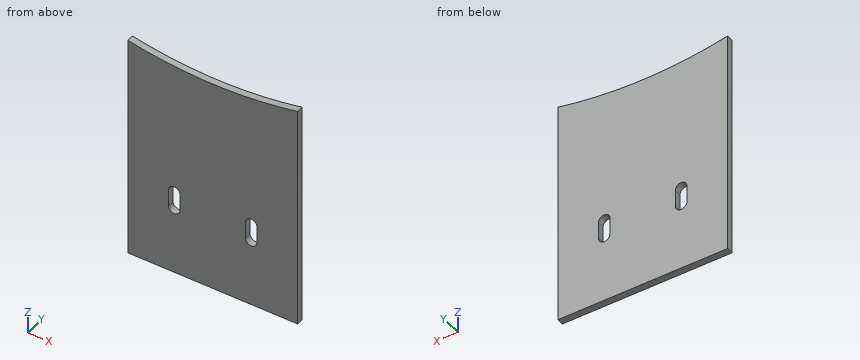
```python
from build123d import *

# Parameters (mm, degrees)
SM_BASE_FLANGE_1_DEPTH = 16


# Sheet-metal steps are written as plain solids
with BuildPart() as part:
    # Sketch 1 → 基体-法兰1 (new body)
    with BuildSketch(Plane(origin=(0, 0, 0), x_dir=(1, 0, 0), z_dir=(0, 1, 0))):
        with BuildLine():
            Line((-200, 964.992357483), (-200, 1497.5))
            Line((-200, 1497.5), (200, 1497.5))
            Line((200, 1497.5), (200, 964.992357483))
            ThreePointArc((200, 964.992357483), (0, 985.5), (-200, 964.992357483))
        make_face()
        with BuildLine():
            Line((-77, 1337), (-77, 1297))
            ThreePointArc((-77, 1297), (-90.5, 1283.5), (-104, 1297))
            Line((-104, 1297), (-104, 1337))
            ThreePointArc((-104, 1337), (-90.5, 1350.5), (-77, 1337))
        make_face(mode=Mode.SUBTRACT)
        with BuildLine():
            Line((77, 1297), (77, 1337))
            ThreePointArc((77, 1337), (90.5, 1350.5), (104, 1337))
            Line((104, 1337), (104, 1297))
            ThreePointArc((104, 1297), (90.5, 1283.5), (77, 1297))
        make_face(mode=Mode.SUBTRACT)
    extrude(amount=SM_BASE_FLANGE_1_DEPTH)


solid = part.part
```
Here's how the part is built. I have some questions about the finished solid (model axes, mm). Round coordinates to 2 decimals unless told otherwise and drop trailing zeros. Write each loop counter-clockwise with the first axis right and the second up, starting at its lowest first coordinate (ties: lowest second). Pieces come first, ordered by that corner, then holes. Notation, with made-up numbers: M 27,86.25 L 69,86.25 A11 cw 69,106.25 Z; hole C -21.5,13.5 d7. An arc over 180 degrees is marked long. Answer as CSV lines item,"result". Start each with the question number.
1. Suppose I cut it at B-B on x = 90.5. Write out the boundary of the cut face in (y, z), then the cut area to 3 significant figures.
2. I need wall thicknesses on probe 1 along X at (y, z) = (13.5, -1300.5); probe 2 along Z at (x, y) = (-13, 2); probe 3 along Z at (x, y) = (93, 6.75). Which ranges of each line are inside material? Lowest first, please.
3. Suppose I cut it at A-A on y = 3. Write out the boundary of the cut face in (x, z).
4. Suppose I cut it at C-C on x = 19. Write out the boundary of the cut face in (y, z), then the cut area to 3 significant figures.
Check result:
1,outline,"M 0,-1497.5 L 16,-1497.5 L 16,-1350.5 L 0,-1350.5 Z; M 0,-1283.5 L 16,-1283.5 L 16,-981.34 L 0,-981.34 Z"
1,area,"7,190 mm2"
2,probe 1,"x = -200 to -104, -77 to 77, 104 to 200"
2,probe 2,"z = -1497.5 to -985.41"
2,probe 3,"z = -1497.5 to -1350.27, -1283.73 to -981.1"
3,outline,"M -200,-1497.5 L 200,-1497.5 L 200,-964.99 A985.5 cw -200,-964.99 Z; hole M -104,-1337 A13.5 ccw -77,-1337 L -77,-1297 A13.5 ccw -104,-1297 Z; hole M 77,-1337 A13.5 ccw 104,-1337 L 104,-1297 A13.5 ccw 77,-1297 Z"
4,outline,"M 0,-1497.5 L 16,-1497.5 L 16,-985.32 L 0,-985.32 Z"
4,area,"8,190 mm2"
